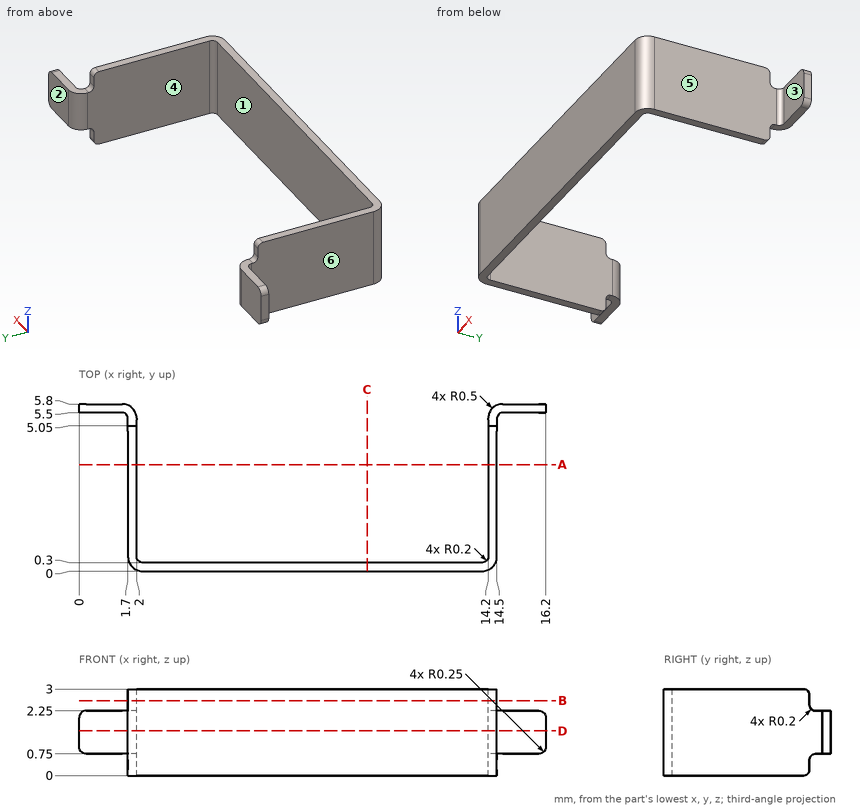
Check sheet for the drawn part. Datum: minimum x, y, z corner. Units: mm. A direction names the side the tool comes from. Coordinates: 2 decimals unless noted, no trailing zeros. Loops run counter-clockwise (first coordinate to the right, second up) from the corner with the lowest first, then second, coordinate; pieces in that order, holes last. Notation, with made-up numbers: (-37.5, 79.25) -> (-5.5, 79.25) arc R23 cw to (-5.5, 99.25) -> close; hole circle Ø9 at (55, -4.5). An arc over 180 degrees is marked (long way). Answer as a JSON object with one key per item and string values. Group by question number.
Item 1: Tool access check on the marked faces 1 and 2. Record the directions out of +Z, -Z, +X, -X, +Y, -Y that give a thin tool (end or side, any length) a straight path to the whole face; none if there is none.
Item 2: Sectioned sample at B-B on z = 2.6. Record the boundary of the cut face in (x, y).
Item 3: Scan lines: probe 1 along X at (y, z) = (3.75, 0.4); probe 2 along Y at (x, z) = (4.5, 2.55). Record each from-to range of solid material in increasing order.
Item 4: Sectioned sample at C-C on x = 10. Record the boundary of the cut face in (y, z), plus the area to 3 significant figures.
Item 5: Depth check by flat-ended pin: pin 1 (0.9 mm diameter, centred on y = 3, z = 2, fed in from +X); pin 2 (1.6 mm diameter, centred on x = 15, z = 1.5, fed in from -Y); pin 3 (1.5 mm diameter, centred on y = 4, z = 1.5, fed in from -X). Enter the tip coordinate at first touch or a pass-through.
Item 6: Mould release check, pull along X, two halves, no side actions. Record for the marked faces 3, 4, 5 and 6: +X half, -X half, draft (parallel to the pull), parting line (faces both ways), or undercut.
Item 7: Sectioned sample at A-A on y = 3.7. Record the boundary of the cut face in (x, z).
Item 8: Sectioned sample at D-D on z = 1.55. Record the boundary of the cut face in (x, y), plus the area to 3 significant figures.
Evaluation:
{
 "1": {"face 1": "+Z, -Z, +Y", "face 2": "+Z, -Z, +X, -X, +Y"},
 "2": {"outline": "(1.7, 0.5) arc R0.5 ccw to (2.2, 0) -> (14, 0) arc R0.5 ccw to (14.5, 0.5) -> (14.5, 5.05) -> (14.2, 5.05) -> (14.2, 0.5) arc R0.2 cw to (14, 0.3) -> (2.2, 0.3) arc R0.2 cw to (2, 0.5) -> (2, 5.05) -> (1.7, 5.05) -> close"},
 "3": {"probe 1": "x = 1.7 to 2, 14.2 to 14.5", "probe 2": "y = 0 to 0.3"},
 "4": {"outline": "(0, 0) -> (0.3, 0) -> (0.3, 3) -> (0, 3) -> close", "area": "0.900 mm²"},
 "5": {"pin 1": "stops at x = 14.5", "pin 2": "stops at y = 0.04", "pin 3": "stops at x = 1.7"},
 "6": {"face 3": "draft", "face 4": "undercut", "face 5": "+X half", "face 6": "-X half"},
 "7": {"outline": "(1.7, 0) -> (2, 0) -> (2, 3) -> (1.7, 3) -> close; (14.2, 0) -> (14.5, 0) -> (14.5, 3) -> (14.2, 3) -> close"},
 "8": {"outline": "(0, 5.5) -> (1.5, 5.5) arc R0.2 cw to (1.7, 5.3) -> (1.7, 0.5) arc R0.5 ccw to (2.2, 0) -> (14, 0) arc R0.5 ccw to (14.5, 0.5) -> (14.5, 5.3) arc R0.2 cw to (14.7, 5.5) -> (16.2, 5.5) -> (16.2, 5.8) -> (14.7, 5.8) arc R0.5 ccw to (14.2, 5.3) -> (14.2, 0.5) arc R0.2 cw to (14, 0.3) -> (2.2, 0.3) arc R0.2 cw to (2, 0.5) -> (2, 5.3) arc R0.5 ccw to (1.5, 5.8) -> (0, 5.8) -> close", "area": "7.98 mm²"}
}
